```python
from build123d import *

# Parameters (mm, degrees)
CROQUIS1_W              = 60
CROQUIS1_H              = 20
SALIENTE_EXTRUIR1_DEPTH = 30
CROQUIS2_W              = 20
CROQUIS2_H              = 20
CORTAR_EXTRUIR1_DEPTH   = 5
CROQUIS4_W              = 20
CROQUIS4_H              = 20
SALIENTE_EXTRUIR2_DEPTH = 20


with BuildPart() as part:
    # Croquis1 → Saliente-Extruir1 (new body)
    with BuildSketch(Plane.XY):
        Rectangle(CROQUIS1_W, CROQUIS1_H)
    extrude(amount=SALIENTE_EXTRUIR1_DEPTH)

    # Croquis2 → Cortar-Extruir1 (cut)
    with BuildSketch(Plane.XY.offset(30)):
        Rectangle(CROQUIS2_W, CROQUIS2_H)
    extrude(amount=-CORTAR_EXTRUIR1_DEPTH, mode=Mode.SUBTRACT)

    # Croquis4 → Saliente-Extruir2 (add)
    with BuildSketch(Plane.XY.offset(30)):
        with Locations((-20, 0)):
            Rectangle(CROQUIS4_W, CROQUIS4_H)
        with Locations((20, 0)):
            Rectangle(CROQUIS4_W, CROQUIS4_H)
    extrude(amount=SALIENTE_EXTRUIR2_DEPTH)


solid = part.part
```
Here's how the part is built. I have some questions about the finished solid (model axes, mm). A direction names the side the tool comes from. Coordinates: 2 decimals unless noted, no trailing zeros. Loops run counter-clockwise (first coordinate to the right, second up) from the corner with the lowest first, then second, coordinate; pieces in that order, holes last. Notation, with made-up numbers: (7, -35.75) - (11, -35.75) arc R15 ccw to (11, -8.75) - close; hole circle Ø3 at (-21.5, 60.25). An arc over 180 degrees is marked (long way). Return JSON: item names as keys, results as strings. Group by question number.
Item 1: On a 3-axis mill with a long thin cutter (end or side, diameter ignored), from which of +Z, -Z, +X, -X, +Y, -Y can I reach the whole of each face in a straight line? I mean faces 1 (the face through (-20, 0, 50)), 2 (the face through (-10, 0, 37)). Say none if no direction works.
Item 2: If we section it at B-B on y = 3.5: Write out the boundary of the cut face in (x, z).
Item 3: Will this pin go through, and if not, where does the flat tip stop? P1, Ø6, axis at x = 4.5, y = 4, coming from the +Z side.
Item 4: If we section it at C-C on x = 0: Write out the boundary of the cut face in (y, z).
Item 5: If we section it at A-A on z = 35.5: Write out the boundary of the cut face in (x, y).
Item 6: I need wall thicknesses on line 1 (X direction, y = 4.25, z = 47.5); line 2 (Z direction, x = 7, y = -3). Which ranges of each line are inside material? Lowest first, please. Write a range as from..to.
Calculated:
{
 "1": {"face 1": "+Z, +X, -X, +Y, -Y", "face 2": "+Z, +Y, -Y"},
 "2": {"outline": "(-30, 0) - (30, 0) - (30, 50) - (10, 50) - (10, 25) - (-10, 25) - (-10, 50) - (-30, 50) - close"},
 "3": {"P1": "stops at z = 25"},
 "4": {"outline": "(-10, 0) - (10, 0) - (10, 25) - (-10, 25) - close"},
 "5": {"outline": "(-30, -10) - (-10, -10) - (-10, 10) - (-30, 10) - close; (10, -10) - (30, -10) - (30, 10) - (10, 10) - close"},
 "6": {"line 1": "x = -30..-10, 10..30", "line 2": "z = 0..25"}
}
